Geometry check sheet. Reference: the model listing, model coordinates, mm. Face numbers are marked on the shaded views. Coordinates: 2 decimals unless noted, no trailing zeros. Write each loop counter-clockwise with the first axis right and the second up, starting at its lowest first coordinate (ties: lowest second). Pieces come first, ordered by that corner, then holes. Notation, with made-up numbers: (-10, 6.25) -> (5, 6.25) arc R23 ccw to (5, 25.25) -> close; hole circle Ø8 at (37, 68.25). An arc over 180 degrees is marked (long way). Use a Markdown table: item, result.
```python
from build123d import *

# Parameters (mm, degrees)
SKETCH_1_W           = 72.3
SKETCH_1_H           = 10
SKETCH_1_R           = 1.4
EXTRUDE_1_DEPTH      = 3
SKETCH_2_W           = 3
SKETCH_2_H           = 14
EXTRUDE_2_DEPTH      = 19
CUT_EXTRUDE_1_REACH  = 77.082
SKETCH_3_R           = 1.65
EXTRUDE_3_DEPTH      = 2
EXTRUDE_3_DEPTH_BACK = 2


with BuildPart() as part:
    # 草图1 → 凸台-拉伸1 (new body)
    with BuildSketch(Plane(origin=(0, 0, 0), x_dir=(1, 0, 0), z_dir=(0, 1, 0))):
        Rectangle(SKETCH_1_W, SKETCH_1_H)
        with Locations(Location((-14.73, 0, 0), (0, 0, 270))):
            Circle(SKETCH_1_R, mode=Mode.SUBTRACT)
        with Locations(Location((14.73, 0, 0), (0, 0, 270))):
            Circle(SKETCH_1_R, mode=Mode.SUBTRACT)
    extrude(amount=EXTRUDE_1_DEPTH)

    # 草图2 → 凸台-拉伸2 (add)
    with BuildSketch(Plane(origin=(0, 0, 0), x_dir=(1, 0, 0), z_dir=(0, 1, 0))):
        with Locations((-34.65, 0)):
            Rectangle(SKETCH_2_W, SKETCH_2_H)
        with Locations((34.65, 0)):
            Rectangle(SKETCH_2_W, SKETCH_2_H)
    extrude(amount=EXTRUDE_2_DEPTH)

    # 切除-拉伸1: up to this face of the body (flat: up to its plane)
    cut_extrude_1_end = Plane(part.part.faces().sort_by_distance((36.15, 9.5, 0))[0])
    # 草图3 → 切除-拉伸1 (cut, up to the picked face)
    with BuildSketch(Plane.ZY.offset(36.15), mode=Mode.PRIVATE) as cut_extrude_1_sk1:
        with Locations((0, 14)):
            Circle(SKETCH_3_R)
    cut_extrude_1_tool1 = split(extrude(cut_extrude_1_sk1.sketch, amount=-CUT_EXTRUDE_1_REACH, mode=Mode.PRIVATE), bisect_by=cut_extrude_1_end, keep=Keep.BOTH, mode=Mode.PRIVATE)
    add(cut_extrude_1_tool1.solids().sort_by(Axis((-36.15, 14, 0), (1, 0, 0)))[0], mode=Mode.SUBTRACT)

    # 草图4 → 凸台-拉伸3 (add, two sides: drawn at the far end of the back side and taken through both)
    with BuildSketch(Plane.XY.offset(-EXTRUDE_3_DEPTH_BACK)):
        Polygon((-36.15, 9), (-24.15, 3), (-36.15, 3), align=None)
        Polygon((36.15, 9), (24.15, 3), (36.15, 3), align=None)
    extrude(amount=EXTRUDE_3_DEPTH + EXTRUDE_3_DEPTH_BACK)


solid = part.part
```
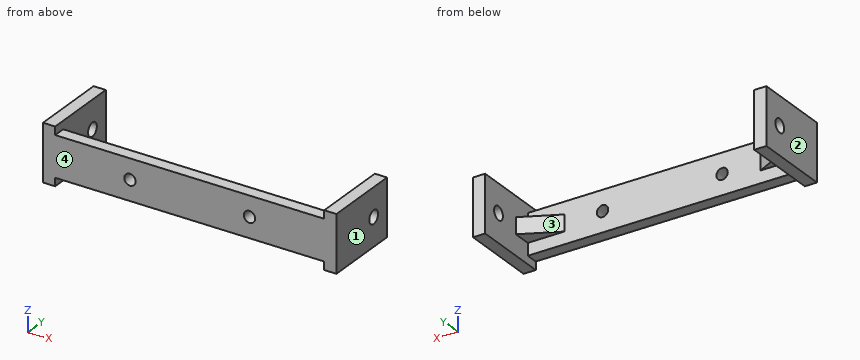
Item 1: Section check B-B on y = 14. Record the boundary of the cut face in (x, z).
Answer block:
| item | result |
|---|---|
| outline | (-36.15, -7) -> (-33.15, -7) -> (-33.15, -1.65) -> (-36.15, -1.65) -> close; (-36.15, 1.65) -> (-33.15, 1.65) -> (-33.15, 7) -> (-36.15, 7) -> close; (33.15, -7) -> (36.15, -7) -> (36.15, -1.65) -> (33.15, -1.65) -> close; (33.15, 1.65) -> (36.15, 1.65) -> (36.15, 7) -> (33.15, 7) -> close |
Item 2: Section check C-C on x = -14.73. Record the boundary of the cut face in (y, z).
Answer block:
| item | result |
|---|---|
| outline | (0, -5) -> (3, -5) -> (3, -1.4) -> (0, -1.4) -> close; (0, 1.4) -> (3, 1.4) -> (3, 5) -> (0, 5) -> close |
Item 3: Section check D-D on z = -6. Record the boundary of the cut face in (x, y).
Answer block:
| item | result |
|---|---|
| outline | (-36.15, 0) -> (-33.15, 0) -> (-33.15, 19) -> (-36.15, 19) -> close; (33.15, 0) -> (36.15, 0) -> (36.15, 19) -> (33.15, 19) -> close |
Item 4: Mould release check, pull along X, two halves, no side actions. Record for the marked faces 1, 2, 3 and 4: +X half, -X half, draft (parallel to the pull), parting line (faces both ways), or undercut.
Answer block:
| item | result |
|---|---|
| face 1 | +X half |
| face 2 | -X half |
| face 3 | undercut |
| face 4 | draft |
Item 5: Thickness scan on L1, parallel to X at y = 2.25, z = 0; L2, parallel to Y at x = 34.8, z = 0; L3, parallel to X at y = 9.25, z = -3. Record the ranges inside material, lowest first. Write a range as [from, to].
Answer block:
| item | result |
|---|---|
| L1 | x = [-36.15, -16.13], [-13.33, 13.33], [16.13, 36.15] |
| L2 | y = [0, 12.35], [15.65, 19] |
| L3 | x = [-36.15, -33.15], [33.15, 36.15] |
Item 6: Section check A-A on z = 0. Record the boundary of the cut face in (x, y).
Answer block:
| item | result |
|---|---|
| outline | (-36.15, 0) -> (-16.13, 0) -> (-16.13, 3) -> (-24.15, 3) -> (-33.15, 7.5) -> (-33.15, 12.35) -> (-36.15, 12.35) -> close; (-36.15, 15.65) -> (-33.15, 15.65) -> (-33.15, 19) -> (-36.15, 19) -> close; (-13.33, 0) -> (13.33, 0) -> (13.33, 3) -> (-13.33, 3) -> close; (16.13, 0) -> (36.15, 0) -> (36.15, 12.35) -> (33.15, 12.35) -> (33.15, 7.5) -> (24.15, 3) -> (16.13, 3) -> close; (33.15, 15.65) -> (36.15, 15.65) -> (36.15, 19) -> (33.15, 19) -> close |
Item 7: Depth check by flat-ended pin: P1, Ø0.9, axis at x = -1, y = 2, coming from the +Z side; P2, Ø4, axis at x = 9.5, z = -1.5, coming from the +Y side; P3, Ø3.5, axis at x = 28.5, y = 6, coming from the -Z side. Enter the tip coordinate at first touch or a pass-through.
Answer block:
| item | result |
|---|---|
| P1 | stops at z = 5 |
| P2 | stops at y = 3 |
| P3 | stops at z = -2 |
